Check sheet for the drawn part. Datum: minimum x, y, z corner. Units: mm. A direction names the side the tool comes from. Give positions to 0.01 mm unless a question says otherwise; leave off trailing zeros. Write each loop counter-clockwise with the first axis right and the second up, starting at its lowest first coordinate (ties: lowest second). Pieces come first, ordered by that corner, then holes. Notation, with made-up numbers: (25.5, -2.5) - (71.5, -2.5) arc R18 cw to (71.5, 28.5) - close; hole circle Ø7 at (15, 15). An arc over 180 degrees is marked (long way). Answer as a JSON object with one key per item and string values. Group by question number.
Item 1: Sectioned sample at C-C, the plane x = 11. Record the boundary of the cut face in (y, z).
Item 2: Sectioned sample at D-D, the plane y = 9. Record the boundary of the cut face in (x, z), and give its area (3 significant figures).
Item 3: Draft check along X on the marked faces 5, 6, 7 and 8. Enter one of: +X half, -X half, draft (parallel to the pull), parting line (faces both ways), or undercut.
Item 4: Tool access check on the marked faces 1, 2, 3 and 4. Record the directions out of +Z, -Z, +X, -X, +Y, -Y that give a thin tool (end or side, any length) a straight path to the whole face; none if there is none.
Item 5: Scan lines: line 1 along Z through (x, y) = (9.05, 8.05); line 2 along Y through (x, z) = (7.75, 13). Record each from-to range of solid material in increasing order. Write a range as [from, to].
Item 6: Go/stop test with flat-tipped pins: pin 1 (4 mm diameter, centred on x = 15.5, y = 2, fed in from -Z); pin 2 (1 mm diameter, centred on x = 10.5, y = 1.5, fed in from -Z) (1 decimal); pin 3 (4.5 mm diameter, centred on x = 5.5, z = 8, fed in from +Y). Record where each tip stops, or that it passes through.
Item 7: Sectioned sample at A-A, the plane y = 4. Record the boundary of the cut face in (x, z).
Item 8: Sectioned sample at B-B, the plane z = 9.05. Record the boundary of the cut face in (x, y).
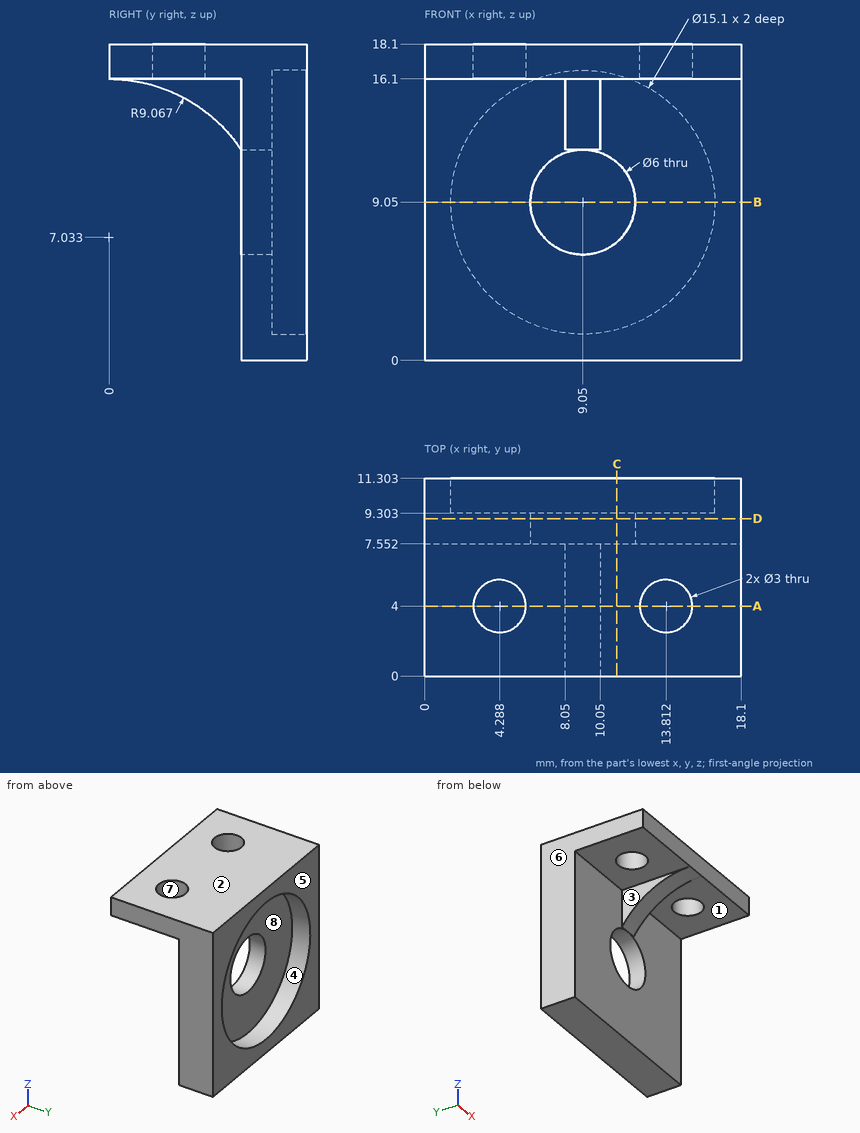
Geometry check:
{
 "1": {"outline": "(0, 16.1) - (7.55, 16.1) - (7.55, 11.33) - (9.3, 11.33) - (9.3, 16.34) - (11.3, 16.34) - (11.3, 18.1) - (0, 18.1) - close; (7.55, 0) - (11.3, 0) - (11.3, 1.76) - (9.3, 1.76) - (9.3, 6.77) - (7.55, 6.77) - close"},
 "2": {"outline": "(0, 0) - (18.1, 0) - (18.1, 18.1) - (0, 18.1) - close; hole circle Ø6 at (9.05, 9.05)", "area": "299 mm^2"},
 "3": {"face 5": "draft", "face 6": "-X half", "face 7": "undercut", "face 8": "undercut"},
 "4": {"face 1": "-Z, +X, -Y", "face 2": "+Z, +X, -X, +Y, -Y", "face 3": "-Z, -X, -Y", "face 4": "+Y"},
 "5": {"line 1": "[0, 6.05], [12.05, 18.1]", "line 2": "[7.55, 9.3]"},
 "6": {"pin 1": "z = 16.1", "pin 2": "z = 15.9", "pin 3": "y = 9.3"},
 "7": {"outline": "(0, 16.1) - (2.79, 16.1) - (2.79, 18.1) - (0, 18.1) - close; (5.79, 16.1) - (8.05, 16.1) - (8.05, 15.17) - (10.05, 15.17) - (10.05, 16.1) - (12.31, 16.1) - (12.31, 18.1) - (5.79, 18.1) - close; (15.31, 16.1) - (18.1, 16.1) - (18.1, 18.1) - (15.31, 18.1) - close"},
 "8": {"outline": "(0, 7.55) - (6.05, 7.55) - (6.05, 9.3) - (1.5, 9.3) - (1.5, 11.3) - (0, 11.3) - close; (12.05, 7.55) - (18.1, 7.55) - (18.1, 11.3) - (16.6, 11.3) - (16.6, 9.3) - (12.05, 9.3) - close"}
}
